Here's the drawing with two shaded views (mm, measured from the low corner). I have some questions. A direction names the side the tool comes from. Coordinates: 2 decimals unless noted, no trailing zeros. Write each loop counter-clockwise with the first axis right and the second up, starting at its lowest first coordinate (ties: lowest second). Pieces come first, ordered by that corner, then holes. Notation, with made-up numbers: (53, -24) -> (93, -24) arc R19 ccw to (93, -18) -> close; hole circle Ø4 at (66, 41.25). An arc over 180 degrees is marked (long way). Use a Markdown table: item, result. Add a question column.
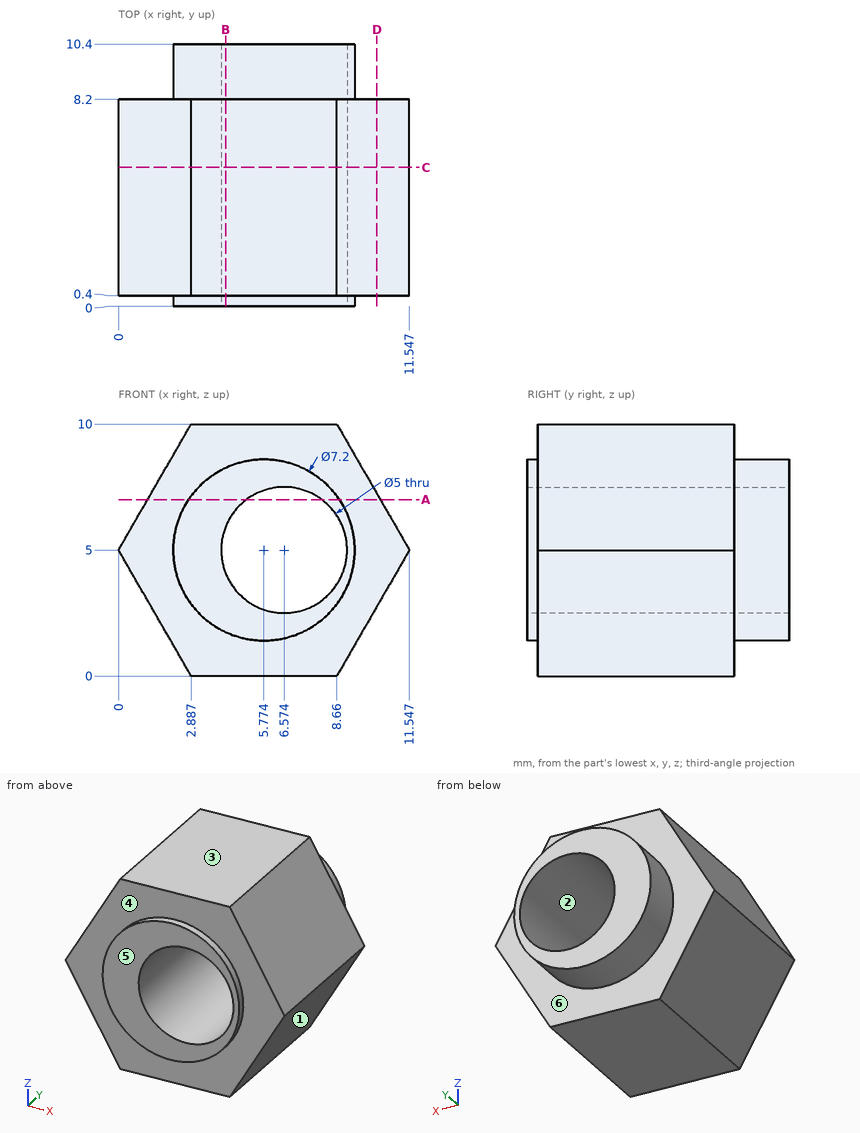
Q1. Which directions (+Z, -Z, +X, -X, +Y, -Y) give clear straight access to the entire face, cutting with the end or side of a thin tool? Please do the marked faces 4, 5 and 6.
Q2. Suppose I cut it at B-B, the plane x = 4.25. Write out the boundary of the cut face in (y, z).
Q3. Thinking about a two-plate mould opening in Z: for the marked faces 1, 2 and 3, which applies, released by +Z, released by -Z, zero draft, split by the parting line, or undercut?
Q4. Will these pins go through, and if not, where does the flat tip stop? pin 1 (3 mm diameter, centred on y = 2.5, z = 8.5, fed in from -X) (1 decimal); pin 2 (1 mm diameter, centred on y = 6.5, z = 1.5, fed in from -X).
Q5. Suppose I cut it at C-C, the plane y = 5.5. Write out the boundary of the cut face in (x, z).
Q6. Suppose I cut it at A-A, the plane z = 7. Write out the boundary of the cut face in (x, y) (1 decimal).
Q7. Suppose I cut it at D-D, the plane x = 10.25. Write out the boundary of the cut face in (y, z).
Q8. Please list where these lines run through material, in increasing order: line 1 (X direction, y = 8.25, z = 5); line 2 (Z direction, x = 7.5, y = 9.25); line 3 (Y direction, x = 3, z = 1.75).
Answer key:
| question | item | result |
|---|---|---|
| 1 | face 4 | -Y |
| 1 | face 5 | +Z, -Z, +X, -X, -Y |
| 1 | face 6 | +Y |
| 2 | outline | (0, 1.74) -> (0.4, 1.74) -> (0.4, 0) -> (8.2, 0) -> (8.2, 1.74) -> (10.4, 1.74) -> (10.4, 4.08) -> (0, 4.08) -> close; (0, 5.92) -> (10.4, 5.92) -> (10.4, 8.26) -> (8.2, 8.26) -> (8.2, 10) -> (0.4, 10) -> (0.4, 8.26) -> (0, 8.26) -> close |
| 3 | face 1 | released by -Z |
| 3 | face 2 | undercut |
| 3 | face 3 | released by +Z |
| 4 | pin 1 | stops at x = 1.2 |
| 4 | pin 2 | stops at x = 1.73 |
| 5 | outline | (0, 5) -> (2.89, 0) -> (8.66, 0) -> (11.55, 5) -> (8.66, 10) -> (2.89, 10) -> close; hole circle Ø5 at (6.57, 5) |
| 6 | outline | (1.2, 0.4) -> (2.8, 0.4) -> (2.8, 0) -> (5.1, 0) -> (5.1, 10.4) -> (2.8, 10.4) -> (2.8, 8.2) -> (1.2, 8.2) -> close; (8.1, 0) -> (8.8, 0) -> (8.8, 0.4) -> (10.4, 0.4) -> (10.4, 8.2) -> (8.8, 8.2) -> (8.8, 10.4) -> (8.1, 10.4) -> close |
| 7 | outline | (0.4, 2.75) -> (8.2, 2.75) -> (8.2, 7.25) -> (0.4, 7.25) -> close |
| 8 | line 1 | x = 2.17 to 4.07, 9.07 to 9.37 |
| 8 | line 2 | z = 1.84 to 2.68, 7.32 to 8.16 |
| 8 | line 3 | y = 0.4 to 8.2 |
